Check sheet for the modelled part. Datum: model origin and axes. Units: mm. A direction names the side the tool comes from. Give positions to 0.01 mm unless a question says otherwise; leave off trailing zeros. Write each loop counter-clockwise with the first axis right and the second up, starting at its lowest first coordinate (ties: lowest second). Pieces come first, ordered by that corner, then holes. Notation, with made-up numbers: (37.25, 71) -> (96.25, 71) arc R26 ccw to (96.25, 88) -> close; hole circle Ø6 at (17, 30.25). An arc over 180 degrees is marked (long way). Return JSON: item names as keys, results as strings.
from build123d import *

# Parameters (mm, degrees)
F1_DEPTH = 9.525
F2_R     = 4.76249
F3_R     = 2.15265
F4_DEPTH = 1.5875


# Not quite as in the source:
# - a fillet or chamfer is up to 0.001 mm smaller than in the source, because OpenCascade refuses the exact size


with BuildPart() as f1:
    # F0 (on Top) → F1 (new body)
    with BuildSketch(Plane.XY):
        with BuildLine():
            Line((-24.257, -28.2194), (-24.257, 0))
            ThreePointArc((-24.257, 0), (0, 24.257), (24.257, 0))
            Line((24.257, 0), (24.257, -28.2194))
            Line((24.257, -28.2194), (35.3695, -28.2194))
            Line((35.3695, -28.2194), (35.3695, -26.6319))
            Line((35.3695, -26.6319), (25.8445, -26.6319))
            Line((25.8445, -26.6319), (25.8445, 0))
            ThreePointArc((25.8445, 0), (0, 25.8445), (-25.8445, 0))
            Line((-25.8445, 0), (-25.8445, -26.6319))
            Line((-25.8445, -26.6319), (-35.3695, -26.6319))
            Line((-35.3695, -26.6319), (-35.3695, -28.2194))
            Line((-35.3695, -28.2194), (-24.257, -28.2194))
        make_face()
    extrude(amount=F1_DEPTH)

    # F2 (radius 4.7625 in the source; OpenCascade refuses exactly that, so slightly less here)
    f2_edges = [f1.edges().sort_by_distance(p)[0] for p in [
        (35.3695, -27.42565, 9.525),
        (35.3695, -27.42565, 0),
        (-35.3695, -27.42565, 0),
        (-35.3695, -27.42565, 9.525),
    ]]
    fillet(f2_edges, radius=F2_R)

    # F3 (on face) → F4 (cut, through all)
    with BuildSketch(Plane.XZ.offset(28.2194)):
        with Locations((30.607, 4.7625)):
            Circle(F3_R)
        with Locations((-30.607, 4.7625)):
            Circle(F3_R)
    extrude(amount=-F4_DEPTH, mode=Mode.SUBTRACT)


solid = f1.part
(1) Depth check by flat-ended pin: pin 1 Ø12 at (x, y) = (-19.5, -9) entering from +Z (3 decimals); pin 2 Ø4 at (y, z) = (20, 5.5) entering from -X; pin 3 Ø5 at (y, z) = (-20, 5) entering from +X; pin 4 Ø1 at (x, z) = (22, 2.5) entering from +Y. Enter the tip coordinate at first touch or a pass-through.
Reply:
{"pin 1": "z = 9.525", "pin 2": "x = -18.55", "pin 3": "x = 25.84", "pin 4": "y = 14.34"}
(2) Cross-section at B-B on z = 5.5. Enter the section's corners in (x, y).
Reply:
{"outline": "(-35.31, -28.22) -> (-32.63, -28.22) -> (-32.63, -26.63) -> (-35.31, -26.63) -> close; (-28.58, -28.22) -> (-24.26, -28.22) -> (-24.26, 0) arc R24.26 cw to (24.26, 0) -> (24.26, -28.22) -> (28.58, -28.22) -> (28.58, -26.63) -> (25.84, -26.63) -> (25.84, 0) arc R25.84 ccw to (-25.84, 0) -> (-25.84, -26.63) -> (-28.58, -26.63) -> close; (32.63, -28.22) -> (35.31, -28.22) -> (35.31, -26.63) -> (32.63, -26.63) -> close"}
(3) Release check for a two-part mould opening along Z. For faces 1 (the flat face through (-21, 13, 0)), 2 (the cylindrical face through (-0.53, 24.25, 4.7)), 3 (the cylindrical face through (28.456, -27.437, 4.857)) record: pulls with the +Z half, pulls with the -Z half, needs draft (parallel to the pull), parting line crosses it, or undercut.
Reply:
{"face 1": "pulls with the -Z half", "face 2": "needs draft", "face 3": "undercut"}
(4) Cross-section at C-C on y = 2. Enter the section's corners in (x, z) (3 decimals), then the cut area to 3 significant figures.
Reply:
{"outline": "(-25.767, 0) -> (-24.174, 0) -> (-24.174, 9.525) -> (-25.767, 9.525) -> close; (24.174, 0) -> (25.767, 0) -> (25.767, 9.525) -> (24.174, 9.525) -> close", "area": "30.3 mm^2"}
(5) Thickness scan on L1, parallel to X at y = -18.5, z = 2.75; L2, parallel to X at y = 6, z = 7.75; L3, parallel to Y at x = -31.5, z = 8.5. Record the ranges inside material, lowest first.
Reply:
{"L1": "-25.84 to -24.26, 24.26 to 25.84", "L2": "-25.14 to -23.5, 23.5 to 25.14", "L3": "-28.22 to -26.63"}
(6) Cross-section at D-D on z = 1.25. Enter the section's corners in (x, y).
Reply:
{"outline": "(-33.82, -28.22) -> (-24.26, -28.22) -> (-24.26, 0) arc R24.26 cw to (24.26, 0) -> (24.26, -28.22) -> (33.82, -28.22) -> (33.82, -26.63) -> (25.84, -26.63) -> (25.84, 0) arc R25.84 ccw to (-25.84, 0) -> (-25.84, -26.63) -> (-33.82, -26.63) -> close"}
(7) Set-up check for faces 4 (the flat face through (24.257, -14, 5)), 5 (the flat face through (-25.844, -13, 5)), 6 (the flat face through (28.6, -26.632, 3.6)): record each of +Z, -Z, +X, -X, +Y, -Y from which the full face is reachable in a straight line by a thin tool's end or side.
Reply:
{"face 4": "+Z, -Z, -Y", "face 5": "+Z, -Z, -X, +Y", "face 6": "+Z, -Z, +X, +Y"}
(8) Cross-section at A-A on y = -18.5. Enter the section's corners in (x, z) (1 decimal), then the cut area to 3 significant figures.
Reply:
{"outline": "(-25.8, 0) -> (-24.3, 0) -> (-24.3, 9.5) -> (-25.8, 9.5) -> close; (24.3, 0) -> (25.8, 0) -> (25.8, 9.5) -> (24.3, 9.5) -> close", "area": "30.2 mm^2"}
